```python
from build123d import *

# Parameters (mm, degrees)
BOSS_EXTRUDE3_DEPTH     = 30
SKETCH3_W               = 108.623523344
SKETCH3_H               = 25
BOSS_EXTRUDE4_DEPTH     = 10
CUT_EXTRUDE2_DEPTH      = 152.009933448
CUT_EXTRUDE2_DEPTH_BACK = 152.009933448
SKETCH5_W               = 108.623523344
SKETCH5_H               = 25
BOSS_EXTRUDE5_DEPTH     = 10
CUT_EXTRUDE3_DEPTH      = 154.310143174
CUT_EXTRUDE3_DEPTH_BACK = 154.310143174
BOSS_EXTRUDE6_DEPTH     = 5
BOSS_EXTRUDE7_DEPTH     = 5
BOSS_EXTRUDE8_DEPTH     = 5
CUT_EXTRUDE4_REACH      = 176.402
SKETCH22_W              = 6.5
SKETCH22_H              = 11.5
SKETCH23_W              = 6.5
SKETCH23_H              = 10
CUT_EXTRUDE5_DEPTH      = 158.671335378


with BuildPart() as part:
    # Sketch1 → Boss-Extrude3 (new body)
    with BuildSketch(Plane(origin=(0, 0, 0), x_dir=(1, 0, 0), z_dir=(0, 1, 0))):
        Polygon((0, -48), (105, -48), (140, -48), (140, -38), (114.68589492, -12.5), (108.623523344, -12.5), (108.623523344, 12.5), (114.68589492, 12.5), (140, 38), (140, 48), (0, 48), align=None)
    extrude(amount=BOSS_EXTRUDE3_DEPTH)

    # Sketch3 → Boss-Extrude4 (add)
    with BuildSketch(Plane(origin=(0, 30, 0), x_dir=(1, 0, 0), z_dir=(0, 1, 0))):
        with Locations((54.311761672, 0)):
            Rectangle(SKETCH3_W, SKETCH3_H)
    extrude(amount=BOSS_EXTRUDE4_DEPTH)

    # Sketch4 → Cut-Extrude2 (cut, two sides: drawn at the far end of the back side and taken through both)
    with BuildSketch(Plane(origin=(0, 30, 0), x_dir=(1, 0, 0), z_dir=(0, 1, 0)).offset(-CUT_EXTRUDE2_DEPTH_BACK)):
        with BuildLine():
            Line((30.5, 34.860728985), (81.5, 34.860728985))
            ThreePointArc((81.5, 34.860728985), (85.860728985, 30.5), (81.5, 26.139271015))
            Line((81.5, 26.139271015), (30.5, 26.139271015))
            ThreePointArc((30.5, 26.139271015), (26.139271015, 30.5), (30.5, 34.860728985))
        make_face()
    extrude(amount=CUT_EXTRUDE2_DEPTH + CUT_EXTRUDE2_DEPTH_BACK, mode=Mode.SUBTRACT)

    # Sketch5 → Boss-Extrude5 (add)
    with BuildSketch(Plane.XZ):
        with Locations((54.311761672, 0)):
            Rectangle(SKETCH5_W, SKETCH5_H)
    extrude(amount=BOSS_EXTRUDE5_DEPTH)

    # Sketch6 → Cut-Extrude3 (cut, two sides: drawn at the far end of the back side and taken through both)
    with BuildSketch(Plane.XZ.offset(-CUT_EXTRUDE3_DEPTH_BACK)):
        with BuildLine():
            Line((30.5, 38.784818055), (80.79497918, 38.784818055))
            ThreePointArc((80.79497918, 38.784818055), (84.804542876, 34.77525436), (80.79497918, 30.765690664))
            Line((80.79497918, 30.765690664), (30.5, 30.765690664))
            ThreePointArc((30.5, 30.765690664), (26.490436304, 34.77525436), (30.5, 38.784818055))
        make_face()
    extrude(amount=CUT_EXTRUDE3_DEPTH + CUT_EXTRUDE3_DEPTH_BACK, mode=Mode.SUBTRACT)

    # Sketch10 → Boss-Extrude6 (add)
    with BuildSketch(Plane(origin=(0, 30, 0), x_dir=(1, 0, 0), z_dir=(0, 1, 0))):
        Polygon((140, 48), (105, 48), (105, 31), (133.051029978, 31), (140, 38), align=None)
    extrude(amount=BOSS_EXTRUDE6_DEPTH)

    # Sketch12 → Boss-Extrude7 (add)
    with BuildSketch(Plane.XZ):
        Polygon((140, 48), (105, 48), (105, 31), (133.051029978, 31), (140, 38), align=None)
        Polygon((105, -48), (105, -31), (133.051029978, -31), (140, -38), (140, -48), align=None)
    extrude(amount=BOSS_EXTRUDE7_DEPTH)

    # Sketch13 → Boss-Extrude8 (add)
    with BuildSketch(Plane(origin=(0, 30, 0), x_dir=(1, 0, 0), z_dir=(0, 1, 0))):
        Polygon((105, -48), (105, -31), (133.051029978, -31), (140, -38), (140, -48), align=None)
    extrude(amount=BOSS_EXTRUDE8_DEPTH)

    # Sketch22 → Cut-Extrude4 (cut, up to next)
    with BuildSketch(Plane(origin=(0, 0, -48), x_dir=(-1, 0, 0), z_dir=(0, 0, -1)), mode=Mode.PRIVATE) as cut_extrude4_sk1:
        with Locations((-3.25, 24.25)):
            Rectangle(SKETCH22_W, SKETCH22_H)
    cut_extrude4_tool1 = extrude(cut_extrude4_sk1.sketch, amount=-CUT_EXTRUDE4_REACH, mode=Mode.PRIVATE) & part.part
    add(cut_extrude4_tool1.solids().sort_by_distance((3.25, 24.25, -48))[0], mode=Mode.SUBTRACT)

    # Sketch23 → Cut-Extrude5 (cut, through all)
    with BuildSketch(Plane(origin=(0, 0, -12.5), x_dir=(-1, 0, 0), z_dir=(0, 0, -1))):
        with Locations((-3.25, 35)):
            Rectangle(SKETCH23_W, SKETCH23_H)
    extrude(amount=-CUT_EXTRUDE5_DEPTH, mode=Mode.SUBTRACT)


solid = part.part
```
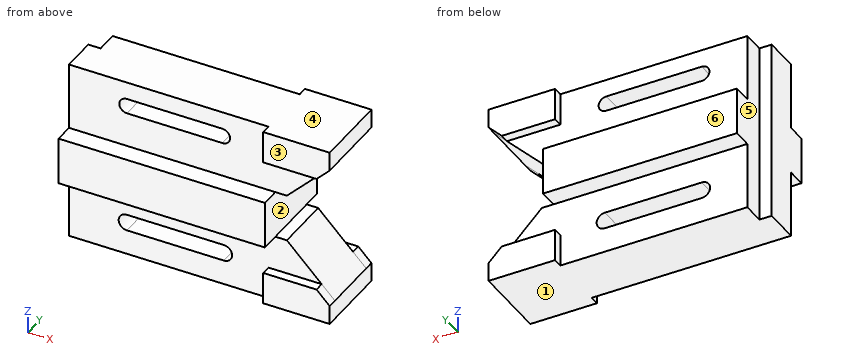
The listing builds one solid part. Answer for the finished solid, in the listing's coordinates (mm). Face numbers are marked on the shaded views. A direction names the side the tool comes from. Give positions to 0.01 mm unless a question says otherwise; leave off trailing zeros. Order: outer loops, then holes, each group sorted by start corner. A loop starts at its lowest first (then second) coordinate and runs counter-clockwise, first axis right, second up.
Item 1: For a pull along Z with two mould halves and no side action, classify the marked faces 1, 2, 3 and 4 as pulls with the +Z half, pulls with the -Z half, needs draft (parallel to the pull), parting line crosses it, or undercut.
From the geometry:
face 1: pulls with the -Z half
face 2: undercut
face 3: needs draft
face 4: pulls with the +Z half
Item 2: The part is cut by section D-D, the plane z = 5. Give the vertices of the cut face in (x, y), and give its area (3 significant figures).
From the geometry:
outline: (0, -10) - (108.62, -10) - (108.62, 40) - (6.5, 40) - (6.5, 18.5) - (0, 18.5) - close
area: 5,290 mm2
Item 3: The part is cut by section C-C, the plane x = 123. Give the vertices of the cut face in (y, z).
From the geometry:
outline: (-5, -48) - (35, -48) - (35, -31) - (30, -31) - (30, -20.88) - (0, -20.88) - (0, -31) - (-5, -31) - close; (-5, 31) - (0, 31) - (0, 20.88) - (30, 20.88) - (30, 31) - (35, 31) - (35, 48) - (-5, 48) - close
Item 4: Given pin 1 Ø2 at (x, z) = (107, 38) entering from -Y; pin 2 Ø13.5 at (x, z) = (127, 40.5) entering from +Y; pin 3 Ø4 at (y, z) = (-3.5, -39.5) entering from -X, each flat-ended and moving along its own axis, determine where each tip first touches the part or whether it passes through.
From the geometry:
pin 1: stops at y = -5
pin 2: stops at y = 35
pin 3: stops at x = 105
Item 5: Which of the six approach directions +Z, -Z, +X, -X, +Y, -Y give full straight-line access (tool end or side, diameter ignored) to the marked faces 5 and 6?
From the geometry:
face 5: +Z, -Z, -X, +Y
face 6: +Z, -Z, +X, -X, +Y
Item 6: Find the intervals of material crossed by probe 1 along Z at (x, y) = (57.5, 4); probe 2 along Z at (x, y) = (126.5, 32.5); probe 3 along Y at (x, z) = (101, -20), in increasing order.
From the geometry:
probe 1: z = -48 to -34.86, -26.14 to 30.77, 38.78 to 48
probe 2: z = -48 to -31, 31 to 48
probe 3: y = 0 to 30
Item 7: The part is cut by section B-B, the plane x = 79. Give the vertices of the cut face in (y, z).
From the geometry:
outline: (-10, -12.5) - (0, -12.5) - (0, -26.14) - (30, -26.14) - (30, -12.5) - (40, -12.5) - (40, 12.5) - (30, 12.5) - (30, 30.77) - (0, 30.77) - (0, 12.5) - (-10, 12.5) - close; (0, -48) - (30, -48) - (30, -34.86) - (0, -34.86) - close; (0, 38.78) - (30, 38.78) - (30, 48) - (0, 48) - close
Item 8: The part is cut by section A-A, the plane y = 23.5. Give the vertices of the cut face in (x, z), and give its area (3 significant figures).
From the geometry:
outline: (6.5, -48) - (140, -48) - (140, -38) - (114.69, -12.5) - (108.62, -12.5) - (108.62, 12.5) - (114.69, 12.5) - (140, 38) - (140, 48) - (6.5, 48) - close; hole (30.5, -34.86) - (81.5, -34.86) arc R4.36 ccw to (81.5, -26.14) - (30.5, -26.14) arc R4.36 ccw to start; hole (30.5, 30.77) - (80.79, 30.77) arc R4.01 ccw to (80.79, 38.78) - (30.5, 38.78) arc R4.01 ccw to start
area: 10,400 mm2
